Here's how the part is built. I have some questions about the finished solid (model axes, mm). Give positions to 0.01 mm unless a question says otherwise; leave off trailing zeros. Order: outer loops, then holes, each group sorted by start corner. A loop starts at its lowest first (then second) coordinate and runs counter-clockwise, first axis right, second up.
from build123d import *

# Parameters (mm, degrees)
PAD015_DEPTH        = 10
REVOLUTION_ANGLE    = -180
REVOLUTION001_ANGLE = 180
PAD014_DEPTH        = 90


with BuildPart() as pad015:
    # Sketch017 → Pad015 (new body)
    with BuildSketch(Plane.XY):
        with BuildLine():
            Line((11.35, -55.552759), (11.35, -59.447241))
            ThreePointArc((8.937894, -60.6), (10.274598, -60.297003), (11.35, -59.447241))
            Line((8.937894, -60.6), (3.062106, -60.6))
            ThreePointArc((0.65, -59.447241), (1.725402, -60.297003), (3.062106, -60.6))
            Line((0.65, -59.447241), (0.65, -55.552759))
            ThreePointArc((3.062106, -54.4), (1.725402, -54.702997), (0.65, -55.552759))
            Line((3.062106, -54.4), (8.937894, -54.4))
            ThreePointArc((11.35, -55.552759), (10.274598, -54.702997), (8.937894, -54.4))
        make_face()
        with BuildLine():
            Line((29.85, -55.552759), (29.85, -59.447241))
            ThreePointArc((27.437894, -60.6), (28.774598, -60.297003), (29.85, -59.447241))
            Line((27.437894, -60.6), (21.562106, -60.6))
            ThreePointArc((19.15, -59.447241), (20.225402, -60.297003), (21.562106, -60.6))
            Line((19.15, -59.447241), (19.15, -55.552759))
            ThreePointArc((21.562106, -54.4), (20.225402, -54.702997), (19.15, -55.552759))
            Line((21.562106, -54.4), (27.437894, -54.4))
            ThreePointArc((29.85, -55.552759), (28.774598, -54.702997), (27.437894, -54.4))
        make_face()
        with BuildLine():
            Line((48.35, -55.552759), (48.35, -59.447241))
            ThreePointArc((45.937894, -60.6), (47.274598, -60.297003), (48.35, -59.447241))
            Line((45.937894, -60.6), (40.062106, -60.6))
            ThreePointArc((37.65, -59.447241), (38.725402, -60.297003), (40.062106, -60.6))
            Line((37.65, -59.447241), (37.65, -55.552759))
            ThreePointArc((40.062106, -54.4), (38.725402, -54.702997), (37.65, -55.552759))
            Line((40.062106, -54.4), (45.937894, -54.4))
            ThreePointArc((48.35, -55.552759), (47.274598, -54.702997), (45.937894, -54.4))
        make_face()
        with BuildLine():
            Line((66.85, -55.552759), (66.85, -59.447241))
            ThreePointArc((64.437894, -60.6), (65.774598, -60.297003), (66.85, -59.447241))
            Line((64.437894, -60.6), (58.562106, -60.6))
            ThreePointArc((56.15, -59.447241), (57.225402, -60.297003), (58.562106, -60.6))
            Line((56.15, -59.447241), (56.15, -55.552759))
            ThreePointArc((58.562106, -54.4), (57.225402, -54.702997), (56.15, -55.552759))
            Line((58.562106, -54.4), (64.437894, -54.4))
            ThreePointArc((66.85, -55.552759), (65.774598, -54.702997), (64.437894, -54.4))
        make_face()
        with BuildLine():
            Line((85.35, -55.552759), (85.35, -59.447241))
            ThreePointArc((82.937894, -60.6), (84.274598, -60.297003), (85.35, -59.447241))
            Line((82.937894, -60.6), (77.062106, -60.6))
            ThreePointArc((74.65, -59.447241), (75.725402, -60.297003), (77.062106, -60.6))
            Line((74.65, -59.447241), (74.65, -55.552759))
            ThreePointArc((77.062106, -54.4), (75.725402, -54.702997), (74.65, -55.552759))
            Line((77.062106, -54.4), (82.937894, -54.4))
            ThreePointArc((85.35, -55.552759), (84.274598, -54.702997), (82.937894, -54.4))
        make_face()
    extrude(amount=PAD015_DEPTH)


with BuildPart() as revolution:
    # Sketch016 → Revolution (revolve)
    with BuildSketch(Plane.YZ.offset(90)):
        with BuildLine():
            ThreePointArc((5.1, 4.5), (3.744276, 5.67641), (2, 6.1))
            Line((2, 6.1), (0, 6.1))
            Line((0, 6.1), (0, 4.5))
            Line((5.1, 4.5), (0, 4.5))
        make_face()
    revolve(axis=Axis((90, 0, 0), (0, 0, 1)), revolution_arc=REVOLUTION_ANGLE)


with BuildPart() as revolution001:
    # Clone2D001 → Revolution001 (revolve)
    with BuildSketch(Plane.YZ):
        with BuildLine():
            ThreePointArc((5.1, 4.5), (3.744276, 5.67641), (2, 6.1))
            Line((2, 6.1), (0, 6.1))
            Line((0, 6.1), (0, 4.5))
            Line((0, 4.5), (5.1, 4.5))
        make_face()
    revolve(axis=Axis((0, 0, 0), (0, 0, 1)), revolution_arc=REVOLUTION001_ANGLE)


with BuildPart() as cut_button_strip:
    # Sketch015 → Pad014 (new body)
    with BuildSketch(Plane.YZ):
        with BuildLine():
            Line((-5.1, 4.5), (5.1, 4.5))
            ThreePointArc((5.1, 4.5), (3.744276, 5.67641), (2, 6.1))
            Line((-2, 6.1), (2, 6.1))
            ThreePointArc((-2, 6.1), (-3.744276, 5.67641), (-5.1, 4.5))
        make_face()
    extrude(amount=PAD014_DEPTH)

    # Fusion002: union Revolution, Revolution001
    add(revolution.part)
    add(revolution001.part)


with BuildPart() as cut_button_strip_1:
    # Fusion002 placement: moved
    add(cut_button_strip.part.moved(Location((-2, -57.3, 0))))

    # Cut002: cut Pad015
    add(pad015.part, mode=Mode.SUBTRACT)


solid = cut_button_strip_1.part
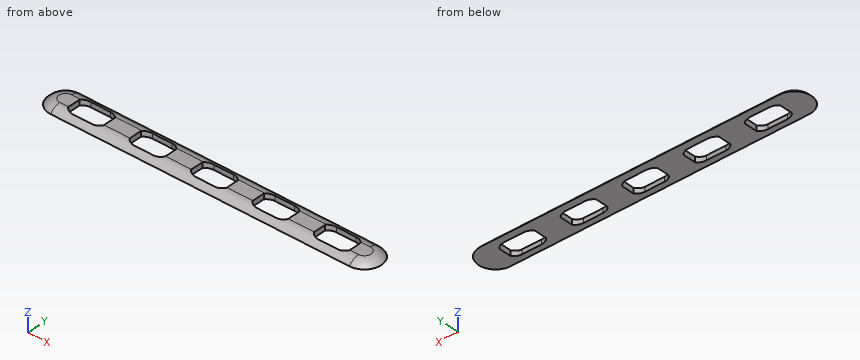
Q1. If we section it at D-D on x = 70: List the corners of the cut face in (y, z) for me.
Filled sheet:
outline: (-62.4, 4.5) - (-52.2, 4.5) arc R3.8 ccw to (-55.3, 6.1) - (-59.3, 6.1) arc R3.8 ccw to start
Q2. If we section it at B-B on z = 5.5: Give the number of separate pieces and of enclosed holes in the cut face, plus the area to 3 significant figures.
Filled sheet:
separate pieces: 1
enclosed holes: 5
area: 466 mm2
Q3. I need wall thicknesses on L1, parallel to X at y = -58, z = 5.7; L2, parallel to X at y = -57.5, z = 4.85; L3, parallel to Y at x = 57, z = 4.7. Which ranges of each line are inside material? Lowest first, please.
Filled sheet:
L1: x = -5.63 to 0.65, 11.35 to 19.15, 29.85 to 37.65, 48.35 to 56.15, 66.85 to 74.65, 85.35 to 91.63
L2: x = -6.81 to 0.65, 11.35 to 19.15, 29.85 to 37.65, 48.35 to 56.15, 66.85 to 74.65, 85.35 to 92.81
L3: y = -62.25 to -60.18, -54.82 to -52.35
Q4. I'm going to push flat-ended pins straight in: P1, Ø0.5, axis at y = -57.5, z = 5.5, coming from the -X side; P2, Ø0.7, axis at x = 5, z = 5.5, coming from the -Y side; P3, Ø0.5, axis at y = -58, z = 5, coming from the +X side; P4, Ø2, axis at x = 40, y = -58, coming from the -Z side. Where does each tip first touch, or does it pass through?
Filled sheet:
P1: stops at x = -6.39
P2: stops at y = -61.81
P3: stops at x = 92.86
P4: passes through
Q5. If we section it at A-A on x = 26: List the corners of the cut face in (y, z) for me, plus the area to 3 significant figures.
Filled sheet:
outline: (-62.4, 4.5) - (-60.6, 4.5) - (-60.6, 5.87) arc R3.8 ccw to start; (-54.4, 4.5) - (-52.2, 4.5) arc R3.8 ccw to (-54.4, 5.99) - close
area: 3.56 mm2
